Input: part model. Units: mm. Frame: model coordinates. Face numbers are marked on the shaded views. A direction names the side the tool comes from. Give positions to 0.01 mm unless a question says otherwise; leave off trailing zeros. Write each loop counter-clockwise with the first axis right and the second up, starting at its lowest first coordinate (ties: lowest second). Pieces come first, ordered by that corner, then holes. Notation, with made-up numbers: (15, 41) -> (69, 41) arc R18 cw to (69, 52) -> close; hole circle Ø5 at (-39, -13.75). An arc over 180 degrees is marked (long way). Answer as a JSON object with one key per item and string values. Group by question number.
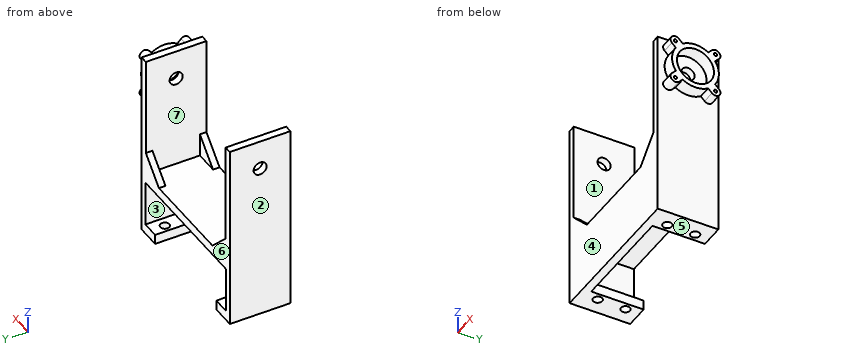
from build123d import *

# Parameters (mm, degrees)
SKETCH1_W            = 95
SKETCH1_H            = 40
BOSS_EXTRUDE1_DEPTH  = 5
SKETCH2_W            = 14.5
SKETCH2_H            = 6
BOSS_EXTRUDE2_DEPTH  = 32
SKETCH4_R            = 2.75
CUT_EXTRUDE1_DEPTH   = 6
BOSS_EXTRUDE5_DEPTH  = 32
SKETCH11_W           = 4.5
SKETCH11_H           = 37
BOSS_EXTRUDE6_DEPTH  = 75
SKETCH12_R           = 4
CUT_EXTRUDE3_DEPTH   = 110
BOSS_EXTRUDE9_DEPTH  = 4
SKETCH16_R           = 11.3
SKETCH16_R_2         = 1
BOSS_EXTRUDE11_DEPTH = 8


with BuildPart() as part:
    # Sketch1 → Boss-Extrude1 (new body)
    with BuildSketch(Plane(origin=(0, 0, 0), x_dir=(1, 0, 0), z_dir=(0, 1, 0))):
        Rectangle(SKETCH1_W, SKETCH1_H)
    extrude(amount=BOSS_EXTRUDE1_DEPTH)

    # Sketch2 → Boss-Extrude2 (add)
    with BuildSketch(Plane(origin=(0, 5, 0), x_dir=(1, 0, 0), z_dir=(0, 1, 0))):
        with Locations((-40.25, 17)):
            Rectangle(SKETCH2_W, SKETCH2_H)
        with Locations((40.25, 17)):
            Rectangle(SKETCH2_W, SKETCH2_H)
    extrude(amount=BOSS_EXTRUDE2_DEPTH)

    # Sketch4 → Cut-Extrude1 (cut)
    with BuildSketch(Plane(origin=(0, 0, -20), x_dir=(-1, 0, 0), z_dir=(0, 0, -1))):
        with Locations((37.5, 11.5)):
            Circle(SKETCH4_R)
        with Locations((37.5, 28.5)):
            Circle(SKETCH4_R)
        with Locations(Location((-37.5, 28.5, 0), (0, 0, 180))):
            Circle(SKETCH4_R)
        with Locations(Location((-37.5, 11.5, 0), (0, 0, 180))):
            Circle(SKETCH4_R)
    extrude(amount=-CUT_EXTRUDE1_DEPTH, mode=Mode.SUBTRACT)

    # Sketch10 → Boss-Extrude5 (add)
    with BuildSketch(Plane(origin=(0, 5, 0), x_dir=(1, 0, 0), z_dir=(0, 1, 0))):
        Polygon((-47.5, -14), (-47.5, -20), (-43.5, -20), (43.5, -20), (47.5, -20), (47.5, -19), (47.5, 14), (43.5, 14), (43.5, -14), (-43.5, -14), (-43.5, 14), (-47.5, 14), align=None)
    extrude(amount=BOSS_EXTRUDE5_DEPTH)

    # Sketch11 → Boss-Extrude6 (add)
    with BuildSketch(Plane.XY.offset(20)):
        with Locations((-45.25, 18.5)):
            Rectangle(SKETCH11_W, SKETCH11_H)
        with Locations((45.25, 18.5)):
            Rectangle(SKETCH11_W, SKETCH11_H)
    extrude(amount=BOSS_EXTRUDE6_DEPTH)

    # Sketch12 → Cut-Extrude3 (cut)
    with BuildSketch(Plane.ZY.offset(47.5)):
        with Locations((77, 18.5)):
            Circle(SKETCH12_R)
    extrude(amount=-CUT_EXTRUDE3_DEPTH, mode=Mode.SUBTRACT)

    # Sketch15 → Boss-Extrude9 (add)
    with BuildSketch(Plane(origin=(0, 37, 0), x_dir=(1, 0, 0), z_dir=(0, 1, 0))):
        Polygon((28.857864376, -20), (43, -34.142135624), (43, -20), align=None)
        Polygon((-28.857864376, -20), (-43, -20), (-43, -34.142135624), align=None)
    boss_extrude9 = extrude(amount=-BOSS_EXTRUDE9_DEPTH)

    # Mirror2: Boss-Extrude9 across plane
    add(boss_extrude9.mirror(Plane.ZX.offset(18.5)))

    # Sketch16 → Boss-Extrude11 (add)
    with BuildSketch(Plane(origin=(47.5, 0, 0), x_dir=(0, 0, -1), z_dir=(1, 0, 0))):
        with BuildLine():
            Line((-66.888373029, 4.145732342), (-69.234713241, 6.492072554))
            ThreePointArc((-69.234713241, 6.492072554), (-77, 4.2), (-84.765286759, 6.492072554))
            Line((-84.765286759, 6.492072554), (-87.111626971, 4.145732342))
            ThreePointArc((-87.111626971, 4.145732342), (-91.354267658, 4.145732342), (-91.354267658, 8.388373029))
            Line((-91.354267658, 8.388373029), (-89.007927446, 10.734713241))
            ThreePointArc((-89.007927446, 10.734713241), (-91.3, 18.5), (-89.007927446, 26.265286759))
            Line((-89.007927446, 26.265286759), (-91.354267658, 28.611626971))
            ThreePointArc((-91.354267658, 28.611626971), (-91.354267658, 32.854267658), (-87.111626971, 32.854267658))
            Line((-87.111626971, 32.854267658), (-84.765286759, 30.507927446))
            ThreePointArc((-84.765286759, 30.507927446), (-77, 32.8), (-69.234713241, 30.507927446))
            Line((-69.234713241, 30.507927446), (-66.888373029, 32.854267658))
            ThreePointArc((-66.888373029, 32.854267658), (-62.645732342, 32.854267658), (-62.645732342, 28.611626971))
            Line((-62.645732342, 28.611626971), (-64.992072554, 26.265286759))
            ThreePointArc((-64.992072554, 26.265286759), (-62.7, 18.5), (-64.992072554, 10.734713241))
            Line((-64.992072554, 10.734713241), (-62.645732342, 8.388373029))
            ThreePointArc((-62.645732342, 8.388373029), (-62.645732342, 4.145732342), (-66.888373029, 4.145732342))
        make_face()
        with Locations((-77, 18.5)):
            Circle(SKETCH16_R, mode=Mode.SUBTRACT)
        with Locations((-64.767052685, 6.267052685)):
            Circle(SKETCH16_R_2, mode=Mode.SUBTRACT)
        with Locations((-89.232947315, 6.267052685)):
            Circle(SKETCH16_R_2, mode=Mode.SUBTRACT)
        with Locations((-89.232947315, 30.732947315)):
            Circle(SKETCH16_R_2, mode=Mode.SUBTRACT)
        with Locations((-64.767052685, 30.732947315)):
            Circle(SKETCH16_R_2, mode=Mode.SUBTRACT)
    extrude(amount=BOSS_EXTRUDE11_DEPTH)


solid = part.part
1. Line query: line 1 (Y direction, x = 37.5, z = -15.5); line 2 (X direction, y = 29.5, z = -4.5); line 3 (X direction, y = 32, z = 33). Output: solid intervals per line, ascending.
2. Section B-B (z = 46.5). Return the cut outline in (x, y).
3. Section C-C (z = 77). Return the cut outline in (x, y), plus the area to 3 significant figures.
4. Contact query for flat-ended pins moving along their axis: pin 1 Ø2 at (y, z) = (29.5, 50) entering from +X; pin 2 Ø10 at (x, y) = (-34.5, 16) entering from +Z; pin 3 Ø1.5 at (x, y) = (17.5, 26.5) entering from -Z; pin 4 Ø2 at (y, z) = (31, 65) entering from +X. Output: stop coordinate, or through.
5. Section A-A (y = 18.5). State how many separate pieces and enclosed holes the cut face has, plus the area to 3 significant figures.
6. Mould query, pull axis Y, two halves, no side actions, for the marked faces 4, 5, 6 and 7. Classes: pulls with the +Y half, pulls with the -Y half, needs draft (parallel to the pull), parting line crosses it, or undercut.
7. Reachability of the marked faces 1, 2 and 3 from +Z, -Z, +X, -X, +Y, -Y: full face, straight path, thin tool, end or side. Return the list, or none.
8. Section D-D (x = 37.5). Return the cut outline in (y, z).
Working result:
{
 "1": {"line 1": "y = 0 to 8.75, 14.25 to 25.75, 31.25 to 37", "line 2": "x = -47.5 to -43.5, 43.5 to 47.5", "line 3": "x = -47.5 to -43, 43 to 47.5"},
 "2": {"outline": "(-47.5, 0) -> (-43, 0) -> (-43, 37) -> (-47.5, 37) -> close; (43, 0) -> (47.5, 0) -> (47.5, 37) -> (43, 37) -> close"},
 "3": {"outline": "(-47.5, 0) -> (-43, 0) -> (-43, 14.5) -> (-47.5, 14.5) -> close; (-47.5, 22.5) -> (-43, 22.5) -> (-43, 37) -> (-47.5, 37) -> close; (43, 0) -> (47.5, 0) -> (47.5, 4.2) -> (55.5, 4.2) -> (55.5, 7.2) -> (47.5, 7.2) -> (47.5, 14.5) -> (43, 14.5) -> close; (43, 22.5) -> (47.5, 22.5) -> (47.5, 29.8) -> (55.5, 29.8) -> (55.5, 32.8) -> (47.5, 32.8) -> (47.5, 37) -> (43, 37) -> close", "area": "309 mm^2"},
 "4": {"pin 1": "stops at x = 47.5", "pin 2": "stops at z = 20", "pin 3": "stops at z = 14", "pin 4": "stops at x = 55.5"},
 "5": {"separate pieces": "3", "enclosed holes": "0", "area": "1,620 mm^2"},
 "6": {"face 4": "pulls with the -Y half", "face 5": "needs draft", "face 6": "pulls with the +Y half", "face 7": "undercut"},
 "7": {"face 1": "+Z", "face 2": "+Z, -Z, -X, +Y, -Y", "face 3": "+Y"},
 "8": {"outline": "(0, -20) -> (8.75, -20) -> (8.75, -14) -> (5, -14) -> (5, 14) -> (37, 14) -> (37, 28.64) -> (33, 28.64) -> (33, 20) -> (4, 20) -> (4, 28.64) -> (0, 28.64) -> close; (14.25, -20) -> (25.75, -20) -> (25.75, -14) -> (14.25, -14) -> close; (31.25, -20) -> (37, -20) -> (37, -14) -> (31.25, -14) -> close"}
}
